Geometry check sheet. Reference: the model listing, model coordinates, mm. A direction names the side the tool comes from. Round coordinates to 2 decimals unless told otherwise and drop trailing zeros. Order: outer loops, then holes, each group sorted by start corner. A loop starts at its lowest first (then second) coordinate and runs counter-clockwise, first axis right, second up.
(1) Cross-section at B-B on z = -8.5. Enter the section's corners in (x, y), and give its area (3 significant figures).
(2) Thickness scan on L1, parallel to Y at x = -5.5, z = 5; L2, parallel to X at y = 13.5, z = 12.75; L3, parallel to X at y = 19, z = -1.5. Record the ranges inside material, lowest first.
(3) Draft check along Z on faces 1 (the face through (0.66, 10.23, -14.985)), 2 (the face through (-3, 35.3, 3)), 3 (the face through (-7, 20.2, -8.1)). Enter one of: pulls with the +Z half, pulls with the -Z half, needs draft (parallel to the pull), parting line crosses it, or undercut.
(4) Gauge pin test, flat ends, axial feed: P1, Ø4, axis at x = -9.5, z = -9.5, coming from the -Y side; P2, Ø1, axis at x = -1, z = 5, coming from the +Y side; P3, Ø4, axis at x = -5.5, y = 37, coming from the +Z side. Record the tip position at first contact, or that the pin passes through.
(5) Cross-section at A-A on x = 12. Enter the section's corners in (y, z).
(6) Cross-section at C-C on y = 12. Enter the section's corners in (x, z), and give its area (3 significant figures).
(7) Set-up check for faces 4 (the face through (-8.44, 20.23, 9.85)), 5 (the face through (-6, 25.3, -10)), 6 (the face through (12, 25.3, 0)): record each of +Z, -Z, +X, -X, +Y, -Y from which the full face is reachable in a straight line by a thin tool's end or side.
from build123d import *

# Parameters (mm, degrees)
SKETCH_1_R               = 2.5
EXTRUDE_1_DEPTH          = 5
SKETCH_2_R               = 3.5
EXTRUDE_2_DEPTH          = 0.3
SKETCH_3_R               = 15
EXTRUDE_3_DEPTH          = 10
SKETCH_4_R               = 6.35
EXTRUDE_4_DEPTH          = 10
SKETCH_5_R               = 6.35
EXTRUDE_5_DEPTH          = 10
SKETCH_6_R               = 3.5
EXTRUDE_6_DEPTH          = 0.3
SKETCH_7_R               = 3.35
EXTRUDE_7_DEPTH          = 3.7
SKETCH_8_R               = 2.5
EXTRUDE_8_DEPTH          = 3
EXTRUDE_START            = 3.7
SKETCH_9_R               = 3.35
EXTRUDE_9_DEPTH          = 3.7
SKETCH_10_R              = 2.5
EXTRUDE_10_DEPTH         = 5.6
SKETCH_11_R              = 2.5
EXTRUDE_11_DEPTH         = 10
PATTERN_CIRCULAR_1_COUNT = 3


with BuildPart() as part:
    # 草图1 → 凸台-拉伸1 (new body)
    with BuildSketch(Plane(origin=(0, 0, 0), x_dir=(1, 0, 0), z_dir=(0, 1, 0))):
        with Locations(Location((0, 0, 0), (0, 0, 270))):
            Circle(SKETCH_1_R)
    extrude(amount=EXTRUDE_1_DEPTH)

    # 草图2 → 凸台-拉伸2 (add)
    with BuildSketch(Plane(origin=(0, 5, 0), x_dir=(1, 0, 0), z_dir=(0, 1, 0))):
        with Locations(Location((0, 0, 0), (0, 0, 270))):
            Circle(SKETCH_2_R)
    extrude(amount=EXTRUDE_2_DEPTH)

    # 草图3 → 凸台-拉伸3 (add)
    with BuildSketch(Plane(origin=(0, 5.3, 0), x_dir=(1, 0, 0), z_dir=(0, 1, 0))):
        with Locations(Location((0, 0, 0), (0, 0, 270))):
            Circle(SKETCH_3_R)
    extrude(amount=EXTRUDE_3_DEPTH)

    # 草图4 → 凸台-拉伸4 (add)
    with BuildSketch(Plane(origin=(0, 15.3, 0), x_dir=(1, 0, 0), z_dir=(0, 1, 0))):
        with Locations(Location((0, 0, 0), (0, 0, 270))):
            Circle(SKETCH_4_R)
    extrude(amount=EXTRUDE_4_DEPTH)

    # 草图5 → 凸台-拉伸5 (add)
    with BuildSketch(Plane(origin=(0, 25.3, 0), x_dir=(1, 0, 0), z_dir=(0, 1, 0))):
        with Locations(Location((0, 0, 0), (0, 0, 270))):
            Circle(SKETCH_5_R)
    extrude(amount=EXTRUDE_5_DEPTH)

    # 草图6 → 凸台-拉伸6 (add)
    with BuildSketch(Plane(origin=(0, 35.3, 0), x_dir=(1, 0, 0), z_dir=(0, 1, 0))):
        with Locations(Location((0, 0, 0), (0, 0, 270))):
            Circle(SKETCH_6_R)
    extrude(amount=EXTRUDE_6_DEPTH)

    # 草图7 → 凸台-拉伸7 (add)
    with BuildSketch(Plane(origin=(0, 35.6, 0), x_dir=(1, 0, 0), z_dir=(0, 1, 0))):
        with Locations(Location((0, 0, 0), (0, 0, 270))):
            Circle(SKETCH_7_R)
    extrude(amount=EXTRUDE_7_DEPTH)

    # 草图8 → 凸台-拉伸8 (add)
    with BuildSketch(Plane(origin=(0, 39.3, 0), x_dir=(1, 0, 0), z_dir=(0, 1, 0))):
        with Locations(Location((0, 0, 0), (0, 0, 270))):
            Circle(SKETCH_8_R)
    extrude(amount=EXTRUDE_8_DEPTH)

    # 草图9 → 凸台-拉伸9 (add)
    with BuildSketch(Plane(origin=(0, 5, 0), x_dir=(-1, 0, 0), z_dir=(0, -1, 0)).offset(EXTRUDE_START)):
        with Locations(Location((0, 0, 0), (0, 0, 270))):
            Circle(SKETCH_9_R)
    extrude(amount=-EXTRUDE_9_DEPTH)

    # 草图10 → 凸台-拉伸10 (add)
    with BuildSketch(Plane(origin=(0, 42.3, 0), x_dir=(1, 0, 0), z_dir=(0, 1, 0))):
        with Locations(Location((0, 0, 0), (0, 0, 270))):
            Circle(SKETCH_10_R)
    extrude(amount=EXTRUDE_10_DEPTH)

    # 草图11 → 凸台-拉伸11 (add)
    with BuildSketch(Plane(origin=(0, 15.3, 0), x_dir=(1, 0, 0), z_dir=(0, 1, 0))):
        with Locations(Location((12, 0, 0), (0, 0, 270))):
            Circle(SKETCH_11_R)
    extrude_11 = extrude(amount=EXTRUDE_11_DEPTH)

    # 阵列(圆周)1: 凸台-拉伸11 ×3 about axis
    pattern_circular_1_axis = Axis((0, 0, 0), (0, 1, 0))
    for i in range(1, PATTERN_CIRCULAR_1_COUNT):
        add(extrude_11.rotate(pattern_circular_1_axis, i * 360 / PATTERN_CIRCULAR_1_COUNT))


solid = part.part
Found:
1. outline: (-12.36, 5.3) - (12.36, 5.3) - (12.36, 15.3) - (-4.37, 15.3) - (-4.37, 25.3) - (-7.63, 25.3) - (-7.63, 15.3) - (-12.36, 15.3) - close
1. area: 280 mm2
2. L1: y = 5.3 to 15.3
2. L2: x = -7.9 to 7.9
2. L3: x = -6.17 to 6.17, 10 to 14
3. face 1: parting line crosses it
3. face 2: needs draft
3. face 3: undercut
4. P1: stops at y = 5.3
4. P2: stops at y = 35.3
4. P3: stops at z = 4.53
5. outline: (5.3, -9) - (15.3, -9) - (15.3, -2.5) - (25.3, -2.5) - (25.3, 2.5) - (15.3, 2.5) - (15.3, 9) - (5.3, 9) - close
6. outline: circle Ø30 at (0, 0)
6. area: 707 mm2
7. face 4: +Y
7. face 5: -Z, +X, -X, +Y
7. face 6: +Z, -Z, +X, +Y
